Can you work these out from the model? Positions are in its coordinate system, mm. Face numbers are marked on the shaded views. A direction names the side the tool comes from. Give positions to 0.01 mm unless a question says otherwise; leave off trailing zeros. Order: outer loops, then holes, each group sorted by start corner. A loop starts at its lowest first (then second) coordinate and runs counter-clockwise, first axis right, second up. Notation, with made-up numbers: (22.25, 84) -> (30.25, 84) arc R17 ccw to (30.25, 97) -> close; hole circle Ø11 at (2.25, 65). An arc over 180 degrees is marked (long way). Answer as CSV lines item,"result".
```python
from build123d import *

# Parameters (mm, degrees)
F1_DEPTH = 12.7


with BuildPart() as f1:
    # F0 (on Front) → F1 (new body)
    with BuildSketch(Plane.XZ):
        with BuildLine():
            Line((-25.4, 43.994091), (0, 0))
            Line((0, 0), (50.8, 0))
            Line((50.8, 0), (50.8, 12.7))
            Line((50.8, 12.7), (13.682348, 12.7))
            ThreePointArc((13.682348, 12.7), (4.157348, 7.200739), (4.157348, 18.199261))
            Line((4.157348, 18.199261), (-14.401477, 50.344091))
            Line((-14.401477, 50.344091), (-25.4, 43.994091))
        make_face()
    extrude(amount=F1_DEPTH)


solid = f1.part
```
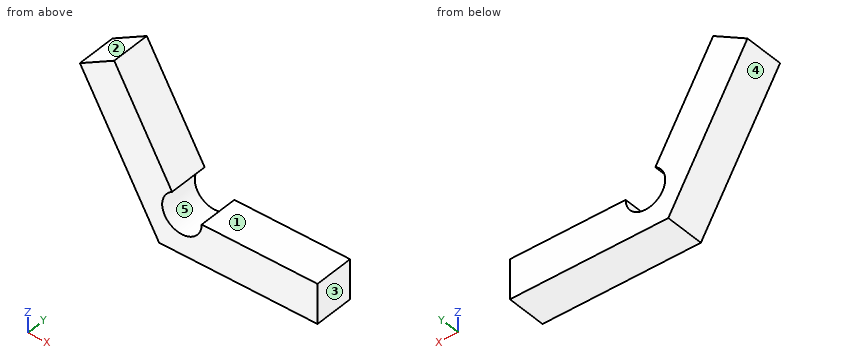
Item 1: Imagine slicing it at B-B, the plane x = -2. Please give me the cut outline in (y, z), then the cut area to 3 significant figures.
Numbers:
outline,"(-12.7, 3.46) -> (0, 3.46) -> (0, 28.86) -> (-12.7, 28.86) -> close"
area,"323 mm²"
Item 2: We'd pull the mould along X, two halves only. Please class the marked faces 3, 4 and 5: released by +X, released by -X, zero draft, split by the parting line, or undercut.
Numbers:
face 3,"released by +X"
face 4,"released by -X"
face 5,"undercut"
Item 3: For pin 1 (1.5 mm diameter, centred on x = 25, z = 13.5, fed in from -Y); pin 2 (3 mm diameter, centred on x = 42.5, y = -2, fed in from +Z); pin 3 (20.5 mm diameter, centred on x = 7.33, z = 12.7, fed in from -Y), each with a flat end and sliding along its axis, tell me the tip position at first contact or that it passes through.
Numbers:
pin 1,"passes through"
pin 2,"stops at z = 12.7"
pin 3,"stops at y = -12.7"
Item 4: Please list where these lines run through material, in increasing order: line 1 along Z through (x, y) = (33, -2); line 2 along X through (y, z) = (-10.5, 10); line 3 along X through (y, z) = (-7.5, 8).
Numbers:
line 1,"z = 0 to 12.7"
line 2,"x = -5.77 to 1.58, 13.08 to 50.8"
line 3,"x = -4.62 to 3.06, 11.6 to 50.8"
Item 5: For the marked faces 1 and 2, which set-ups out of +Z, -Z, +X, -X, +Y, -Y let a thin tool reach every point of the face, with its end or its side?
Numbers:
face 1,"+Z, +X, +Y, -Y"
face 2,"+Z, -X, +Y, -Y"
Item 6: Imagine slicing it at C-C, the plane z = 31. Please give me the cut outline in (x, y), then the cut area to 3 significant figures.
Numbers:
outline,"(-17.9, -12.7) -> (-3.23, -12.7) -> (-3.23, 0) -> (-17.9, 0) -> close"
area,"186 mm²"
Item 7: Imagine slicing it at A-A, the plane y = -2.5. Please give me the cut outline in (x, z).
Numbers:
outline,"(-25.4, 43.99) -> (0, 0) -> (50.8, 0) -> (50.8, 12.7) -> (13.68, 12.7) arc R6.35 cw (long way) to (4.16, 18.2) -> (-14.4, 50.34) -> close"
